```python
from build123d import *

# Parameters (mm, degrees)
SKETCH1_R           = 49.5046
BOSS_EXTRUDE1_DEPTH = 5.08
SKETCH2_R           = 47.625
BOSS_EXTRUDE2_DEPTH = 3.175
SKETCH3_R           = 6.731
SKETCH3_R_2         = 3.96875
SKETCH3_R_3         = 10
SKETCH3_R_4         = 3.175
SKETCH3_R_5         = 2
CUT_EXTRUDE1_DEPTH  = 9.255
SKETCH7_R           = 56.423127019
CUT_EXTRUDE2_DEPTH  = 3.175


with BuildPart() as part:
    # Sketch1 → Boss-Extrude1 (new body)
    with BuildSketch(Plane.XY):
        Circle(SKETCH1_R)
    extrude(amount=BOSS_EXTRUDE1_DEPTH)

    # Sketch2 → Boss-Extrude2 (add)
    with BuildSketch(Plane.XY.offset(5.08)):
        Circle(SKETCH2_R)
    extrude(amount=BOSS_EXTRUDE2_DEPTH)

    # Sketch3 → Cut-Extrude1 (cut, through all)
    with BuildSketch(Plane.XY.offset(8.255)):
        with Locations((-12.7, -31.166793627)):
            Circle(SKETCH3_R)
        with Locations((12.7, -31.166793627)):
            Circle(SKETCH3_R)
        with Locations((-36.83, 0)):
            Circle(SKETCH3_R_2)
        with Locations((36.83, 0)):
            Circle(SKETCH3_R_2)
        with Locations((0, 6.35)):
            Circle(SKETCH3_R_3)
        with Locations((-14.921345457, -10.968575281)):
            Circle(SKETCH3_R_4)
        with Locations((0, 28.326878759)):
            Circle(SKETCH3_R_5)
        with Locations((21.976878759, 6.35)):
            Circle(SKETCH3_R_5)
        with Locations((0, -15.626878759)):
            Circle(SKETCH3_R_5)
        with Locations((-21.976878759, 6.35)):
            Circle(SKETCH3_R_5)
    extrude(amount=-CUT_EXTRUDE1_DEPTH, mode=Mode.SUBTRACT)

    # Sketch7 → Cut-Extrude2 (cut)
    with BuildSketch(Plane.XY.offset(8.255)):
        Circle(SKETCH7_R)
    extrude(amount=-CUT_EXTRUDE2_DEPTH, mode=Mode.SUBTRACT)


solid = part.part
```
Check sheet for the modelled part. Datum: model origin and axes. Units: mm. Coordinates: 2 decimals unless noted, no trailing zeros. Write each loop counter-clockwise with the first axis right and the second up, starting at its lowest first coordinate (ties: lowest second). Pieces come first, ordered by that corner, then holes. Notation, with made-up numbers: M -11.75,-28 L 6.25,-28 A22 cw 6.25,-9 Z; hole C 39.25,89 d5. An arc over 180 degrees is marked long. Use one line per item in the form item = value.
Item 1: Material ranges on L1, parallel to X at y = -36, z = 2.6; L2, parallel to Y at x = -12.7, z = 1.4; L3, parallel to X at y = -2.5, z = 4.3, recorded low to high. Write a range as from..to.
Answer below:
L1 = -33.98..-17.38, -8.02..8.02, 17.38..33.98
L2 = -47.85..-37.9, -24.44..-13.24, -8.7..47.85
L3 = -49.44..-39.91, -33.75..-4.66, 4.66..33.75, 39.91..49.44
Item 2: Sectioned sample at B-B, the plane y = 6.35. Record the cut outline in (x, z).
Answer below:
outline = M -49.1,0 L -23.98,0 L -23.98,5.08 L -49.1,5.08 Z; M -19.98,0 L -10,0 L -10,5.08 L -19.98,5.08 Z; M 10,0 L 19.98,0 L 19.98,5.08 L 10,5.08 Z; M 23.98,0 L 49.1,0 L 49.1,5.08 L 23.98,5.08 Z
Item 3: Release check for a two-part mould opening along Y. For faces 1 (the face through (-6.445, 49.083, 2.504)), 2 (the face through (10, 1, 0)), 3 (the face through (0.923, -17.401, 2.576)), 4 (the face through (-0.434, 26.374, 2.576)) record: pulls with the +Y half, pulls with the -Y half, needs draft (parallel to the pull), parting line crosses it, or undercut.
Answer below:
face_1 = parting line crosses it
face_2 = needs draft
face_3 = undercut
face_4 = undercut
Item 4: Gauge pin test, flat ends, axial feed: pin 1 Ø1.5 at (y, z) = (4, 2.5) entering from +X; pin 2 Ø2 at (y, z) = (31.5, 3) entering from -X; pin 3 Ø1 at (y, z) = (27, 3.5) entering from -X. Record the tip position at first contact, or that the pin passes through.
Answer below:
pin_1 = 49.4
pin_2 = -38.99
pin_3 = -41.81
Item 5: Sectioned sample at A-A, the plane x = 0. Record the cut outline in (y, z), and give its area (3 significant figures).
Answer below:
outline = M -49.5,0 L -17.63,0 L -17.63,5.08 L -49.5,5.08 Z; M -13.63,0 L -3.65,0 L -3.65,5.08 L -13.63,5.08 Z; M 16.35,0 L 26.33,0 L 26.33,5.08 L 16.35,5.08 Z; M 30.33,0 L 49.5,0 L 49.5,5.08 L 30.33,5.08 Z
area = 361 mm^2
Item 6: Sectioned sample at C-C, the plane z = 3.6. State how many separate pieces and enclosed holes the cut face has, and give its area (3 significant figures).
Answer below:
separate_pieces = 1
enclosed_holes = 10
area = 6,920 mm^2
Item 7: Sectioned sample at D-D, the plane x = 34. Record the cut outline in (y, z), and give its area (3 significant figures).
Answer below:
outline = M -35.98,0 L -2.78,0 L -2.78,5.08 L -35.98,5.08 Z; M 2.78,0 L 35.98,0 L 35.98,5.08 L 2.78,5.08 Z
area = 337 mm^2
